```python
from build123d import *

# Parameters (mm, degrees)
BOSS_EXTRUDE1_DEPTH     = 32.2834
CUT_EXTRUDE1_REACH      = 62.594
CUT_EXTRUDE1_END_RADIUS = 32.2707
SKETCH2_R               = 1.9939
BOSS_EXTRUDE2_DEPTH     = 3.175
CUT_EXTRUDE2_DEPTH      = 3.175


with BuildPart() as part:
    # Sketch1 → Boss-Extrude1 (new body)
    with BuildSketch(Plane.XY):
        with BuildLine():
            Line((-36.2585, 36.2585), (-32.2707, 36.2585))
            ThreePointArc((-32.2707, 36.2585), (0, 3.9878), (32.2707, 36.2585))
            Line((32.2707, 36.2585), (36.2585, 36.2585))
            ThreePointArc((36.2585, 36.2585), (0, 0), (-36.2585, 36.2585))
        make_face()
    extrude(amount=-BOSS_EXTRUDE1_DEPTH)

    # Cut-Extrude1: up to this cylinder (the profile starts outside it)
    cut_extrude1_end = Plane(origin=(0, 36.2585, -16.1417), z_dir=(0, 0, 1)) * Cylinder(CUT_EXTRUDE1_END_RADIUS, 190.7294, mode=Mode.PRIVATE)
    # Sketch2 → Cut-Extrude1 (cut, up to the surface)
    with BuildSketch(Plane(origin=(0, 0, 0), x_dir=(1, 0, 0), z_dir=(0, 1, 0)), mode=Mode.PRIVATE) as cut_extrude1_sk1:
        with Locations(Location((0, 16.1417, 0), (0, 0, 90))):
            Circle(SKETCH2_R)
    cut_extrude1_tool1 = extrude(cut_extrude1_sk1.sketch, amount=CUT_EXTRUDE1_REACH, mode=Mode.PRIVATE) - cut_extrude1_end
    add(cut_extrude1_tool1.solids().sort_by_distance((0, 0, -16.1417))[0], mode=Mode.SUBTRACT)

    # Sketch4 → Boss-Extrude2 (add)
    with BuildSketch(Plane.XY.offset(-6.35)):
        with BuildLine():
            Line((-36.2585, 36.2585), (-38.1635, 36.2585))
            ThreePointArc((-38.1635, 36.2585), (-37.555411186, 33.230080338), (-35.825412395, 30.671134883))
            ThreePointArc((-35.825412395, 30.671134883), (-36.150065958, 33.456437642), (-36.2585, 36.2585))
        make_face()
    extrude(amount=-BOSS_EXTRUDE2_DEPTH)

    # Sketch5 → Cut-Extrude2 (cut)
    with BuildSketch(Plane.XY.offset(-6.35)):
        with BuildLine():
            Line((-32.2707, 36.2585), (-34.1757, 36.2585))
            ThreePointArc((-34.1757, 36.2585), (-33.552449463, 33.219498064), (-31.783319989, 30.671134883))
            ThreePointArc((-31.783319989, 30.671134883), (-32.148624099, 33.454209171), (-32.2707, 36.2585))
        make_face()
    extrude(amount=-CUT_EXTRUDE2_DEPTH, mode=Mode.SUBTRACT)


solid = part.part
```
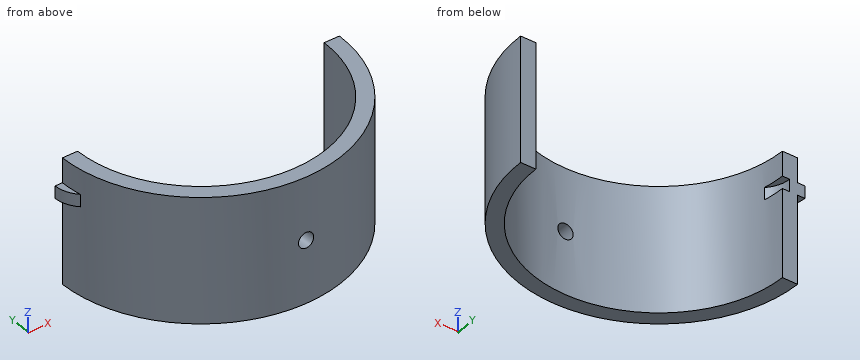
Source: CAD feature listing. Evaluate the final solid. Frame: model axes, mm. Coordinates: 2 decimals unless noted, no trailing zeros. Loops run counter-clockwise (first coordinate to the right, second up) from the corner with the lowest first, then second, coordinate; pieces in that order, holes last. Notation, with made-up numbers: (22, -20) -> (74, -20) arc R19 ccw to (74, -6) -> close; hole circle Ø6 at (36, 26.25). An arc over 180 degrees is marked (long way). One line per item, written item: value. Start each with the question number.
Q1. Section query D-D, the plane y = 32. Return the cut outline in (x, z) (3 decimals).
Q2. Section query B-B, the plane x = 0. Return the cut outline in (y, z).
Q3. Line query: line 1 along X through (y, z) = (34.5, -2); line 2 along X through (y, z) = (8.5, -14.5); line 3 along Y through (x, z) = (-16, -24). Output: solid intervals per line, ascending.
Q4. Contact query for flat-ended pins moving along their axis: P1, Ø8, axis at x = -25, z = -8.5, coming from the -Y side; P2, Ø12, axis at y = 19, z = -12.5, coming from the -X side; P3, Ø12, axis at x = -15, y = 19.5, coming from the +Z side; P4, Ø1.5, axis at y = 18, z = -15.5, coming from the +X side. Output: stop coordinate, or through.
Q5. Section query A-A, the plane y = 12. Return the cut outline in (x, z).
Q6. Section query C-C, the plane z = -11. Return the cut outline in (x, y), and give its area (3 significant figures).
Results:
1. outline: (-36.907, -9.525) -> (-36.008, -9.525) -> (-36.008, -32.283) -> (-31.988, -32.283) -> (-31.988, -9.525) -> (-32.895, -9.525) -> (-32.895, -6.35) -> (-31.988, -6.35) -> (-31.988, 0) -> (-36.008, 0) -> (-36.008, -6.35) -> (-36.907, -6.35) -> close; (31.988, -32.283) -> (36.008, -32.283) -> (36.008, 0) -> (31.988, 0) -> close
2. outline: (0, -32.28) -> (3.99, -32.28) -> (3.99, -18.14) -> (0, -18.14) -> close; (0, -14.15) -> (3.99, -14.15) -> (3.99, 0) -> (0, 0) -> close
3. line 1: -36.22 to -32.22, 32.22 to 36.22
3. line 2: -23.33 to -16.46, 16.46 to 23.33
3. line 3: 3.72 to 8.23
4. P1: y = 6.7
4. P2: x = -34.47
4. P3: through
4. P4: x = 31.75
5. outline: (-26.95, -32.28) -> (-21.28, -32.28) -> (-21.28, 0) -> (-26.95, 0) -> close; (21.28, -32.28) -> (26.95, -32.28) -> (26.95, 0) -> (21.28, 0) -> close
6. outline: (-36.26, 36.26) arc R36.26 ccw to (36.26, 36.26) -> (32.27, 36.26) arc R32.27 cw to (-32.27, 36.26) -> close
6. area: 429 mm^2
